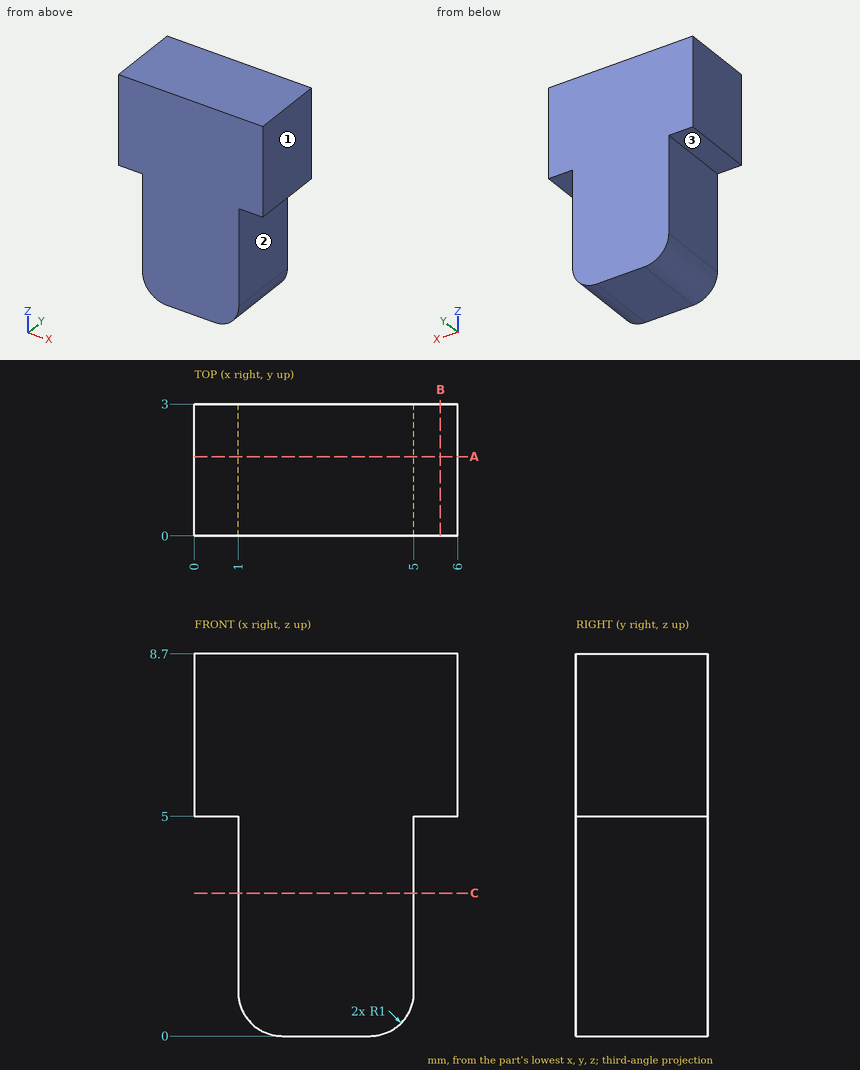
The figure shows three views and two pictorial views of one solid part (mm, origin at its lowest corner). Answer the questions. A direction names the side the tool comes from. Coordinates: 2 decimals unless noted, no trailing zeros. Write each loop counter-clockwise with the first axis right and the second up, starting at its lowest first coordinate (ties: lowest second). Pieces come first, ordered by that corner, then holes. Notation, with made-up numbers: (-9, -32) -> (27, -32) arc R19 ccw to (27, -22) -> close; hole circle Ø10 at (12, 14.25). An arc over 180 degrees is marked (long way). Answer as a JSON object with one key per item and string values.
Q1. Consider line 1 (X direction, y = 0.1, z = 2.75); line 2 (Z direction, x = 0.3, y = 0.1); line 3 (Z direction, x = 4.45, y = 1.8). Determine where each line is inside the solid, lowest interval first. Write a range as [from, to].
The answers:
{"line 1": "x = [1, 5]", "line 2": "z = [5, 8.7]", "line 3": "z = [0.11, 8.7]"}
Q2. The part is cut by section C-C on z = 3.25. Give the vertices of the cut face in (x, y), then the cut area to 3 significant figures.
The answers:
{"outline": "(1, 0) -> (5, 0) -> (5, 3) -> (1, 3) -> close", "area": "12.0 mm2"}
Q3. A tool of negligible diameter and unlimited length cuts with its end or side. For the marked faces 1, 2 and 3, from which of +Z, -Z, +X, -X, +Y, -Y can it reach the whole face along a straight path? Write none if from no direction.
The answers:
{"face 1": "+Z, -Z, +X, +Y, -Y", "face 2": "-Z, +X, +Y, -Y", "face 3": "-Z, -X, +Y, -Y"}
Q4. A flat-ended cylindrical pin translates along its axis: pin 1 Ø1 at (y, z) = (2.5, 4) entering from -X. Find the tip coordinate at first contact, or state that the pin passes through.
The answers:
{"pin 1": "stops at x = 1"}
Q5. The part is cut by section B-B on x = 5.6. Give the vertices of the cut face in (y, z), then the cut area to 3 significant figures.
The answers:
{"outline": "(0, 5) -> (3, 5) -> (3, 8.7) -> (0, 8.7) -> close", "area": "11.1 mm2"}
Q6. The part is cut by section A-A on y = 1.8. Give the vertices of the cut face in (x, z), then the cut area to 3 significant figures.
The answers:
{"outline": "(0, 5) -> (1, 5) -> (1, 1) arc R1 ccw to (2, 0) -> (4, 0) arc R1 ccw to (5, 1) -> (5, 5) -> (6, 5) -> (6, 8.7) -> (0, 8.7) -> close", "area": "41.8 mm2"}
